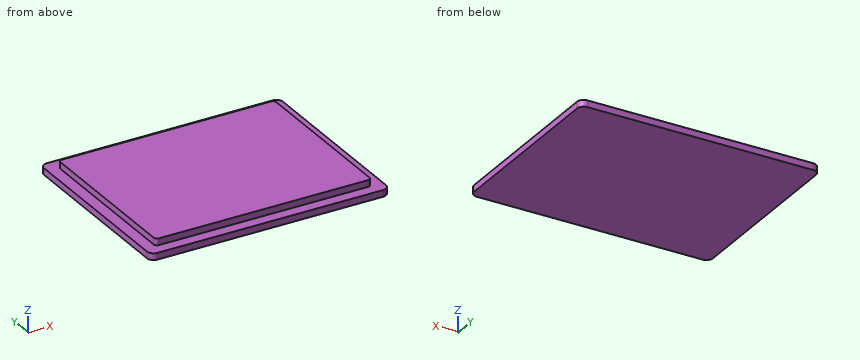
Autodesk Fusion 360 part; units mm, degrees
sketch "Skizze1" plane through (0, 0, 0) normal (0, 0, 1) x (1, 0, 0)
  line L0 (0, 0) -> (18.1, 0)
  line L1 (18.1, 0) -> (18.1, 14.3)
  line L2 (18.1, 14.3) -> (0, 14.3)
  line L3 (0, 14.3) -> (0, 0)
  dimension "d1" = 18.1
  dimension "d2" = 14.3
extrude "Extrusion1" add sketch "Skizze1" along normal blind 2
sketch "Skizze2" plane through (0, 0, 2) normal (0, 0, 1) x (-1, 0, 0)
  line L0 (0, 0) -> (-16.35, 0)
  line L1 (-16.35, 0) -> (-16.35, -12.55)
  line L2 (-16.35, -12.55) -> (0, -12.55)
  line L3 (0, -12.55) -> (0, 0)
  line L4 (0, -14.3) -> (0, 0)
  line L5 (0, 0) -> (-18.1, 0)
  line L6 (-18.1, 0) -> (-18.1, -14.3)
  line L7 (-18.1, -14.3) -> (0, -14.3)
  point P0 (-18.1, 0)
  point P1 (0, -14.3)
  dimension "d19" = 16.35
  dimension "d20" = 12.55
extrude "Extrusion2" cut sketch "Skizze2" against normal blind 1 contours L1 L2 L4 L5 L6 L7
mirror "Spiegeln1" about plane through (0, 14.3, 0) normal (-1, 0, 0) of bodies 1 merged
mirror "Spiegeln2" about plane through (0, 0, 0) normal (0, 1, 0) of bodies 1 merged
fillet "Abrundung1" radius 0.5 4 edges at (-16.35, -12.55, 1.5) (-16.35, 12.55, 1.5) (16.35, 12.55, 1.5) (16.35, -12.55, 1.5)
fillet "Abrundung1" radius 1 4 edges at (-18.1, -14.3, 0.5) (-18.1, 14.3, 0.5) (18.1, 14.3, 0.5) (18.1, -14.3, 0.5)
equation "d1 = ( ( 37.6 - 0.5 ) / 2 ) * 1 mm - 0.45 mm"
equation "d2 = ( ( 30 - 0.5 ) / 2 ) * 1 mm - 0.45 mm"
equation "d19 = ( ( 33.6 - 0.5 ) / 2 ) * 1 mm - 0.2 mm"
equation "d20 = ( ( 26 - 0.5 ) / 2 ) * 1 mm - 0.2 mm"
Model file for the job. Use its own axes, mm. Round coordinates to 2 decimals unless told otherwise and drop trailing zeros. Write each loop counter-clockwise with the first axis right and the second up, starting at its lowest first coordinate (ties: lowest second). Pieces come first, ordered by that corner, then holes. Notation, with made-up numbers: (37, -13.5) - (96, -13.5) arc R30 cw to (96, 12.5) - close; hole circle Ø5 at (25, 54). An arc over 180 degrees is marked (long way). One line per item, written item: value.
(1) Drop flat-ended pins along their axis: P1, Ø0.5, axis at y = 2.5, z = 1.5, coming from the -X side; P2, Ø0.5, axis at x = -7.5, z = 1.5, coming from the +Y side; P3, Ø0.8, axis at x = -5, z = 1.5, coming from the -Y side. Give the stop position or say it passes through.
Values follow:
P1: stops at x = -16.35
P2: stops at y = 12.55
P3: stops at y = -12.55
(2) Wall check: probe 1 along Y at (x, z) = (5.5, 1.1); probe 2 along X at (y, z) = (6, 1.35); probe 3 along Z at (x, y) = (-4.5, -13). Give the ranges that are in metal, low to high.
Values follow:
probe 1: y = -12.55 to 12.55
probe 2: x = -16.35 to 16.35
probe 3: z = 0 to 1
(3) Cut at B-B, the plane y = -5.5. Give the cut face in (x, z), plus the area to 3 significant figures.
Values follow:
outline: (-18.1, 0) - (18.1, 0) - (18.1, 1) - (16.35, 1) - (16.35, 2) - (-16.35, 2) - (-16.35, 1) - (-18.1, 1) - close
area: 68.9 mm²
(4) Cut at A-A, the plane z = 1.6. Give the cut face in (x, y).
Values follow:
outline: (-16.35, -12.05) arc R0.5 ccw to (-15.85, -12.55) - (15.85, -12.55) arc R0.5 ccw to (16.35, -12.05) - (16.35, 12.05) arc R0.5 ccw to (15.85, 12.55) - (-15.85, 12.55) arc R0.5 ccw to (-16.35, 12.05) - close
